from build123d import *

# Parameters (mm, degrees)
F0_R     = 1.25
F1_DEPTH = 0.55
F2_R     = 0.695
F3_DEPTH = 7.3
F4_W     = 0.45
F4_H     = 0.45
F4_H_2   = 0.575
F4_W_2   = 0.575
F5_DEPTH = 0.3
F6_R     = 0.2


with BuildPart() as f1:
    # F0 (on Top) → F1 (new body)
    with BuildSketch(Plane.XY):
        Circle(F0_R)
    extrude(amount=F1_DEPTH)

    # F2 (on face) → F3 (join)
    with BuildSketch(Plane(origin=(0, 0, 0), x_dir=(1, 0, 0), z_dir=(0, 0, -1))):
        Circle(F2_R)
    extrude(amount=F3_DEPTH)

    # F4 (on face) → F5 (cut)
    with BuildSketch(Plane.XY.offset(0.55)):
        Rectangle(F4_W, F4_H)
        with Locations((0, 0.5125)):
            Rectangle(F4_W, F4_H_2)
        with Locations((-0.5125, 0)):
            Rectangle(F4_W_2, F4_H)
        with Locations((0, -0.5125)):
            Rectangle(F4_W, F4_H_2)
        with Locations((0.5125, 0)):
            Rectangle(F4_W_2, F4_H)
    extrude(amount=-F5_DEPTH, mode=Mode.SUBTRACT)

    # F6
    f6_edges = [f1.edges().sort_by_distance(p)[0] for p in [
        (-1.25, 0, 0.55),
        (-1.25, 0, 0),
    ]]
    fillet(f6_edges, radius=F6_R)


solid = f1.part
CAD build for the part. Positions are in the model's coordinates, mm. Round coordinates to 2 decimals unless told otherwise and drop trailing zeros. Write each loop counter-clockwise with the first axis right and the second up, starting at its lowest first coordinate (ties: lowest second). Pieces come first, ordered by that corner, then holes.
(1) Slice it at C-C, the plane z = -2.5. Write the cut outline in (x, y) (3 decimals).
(2) Slice it at A-A, the plane y = 0. Write the cut outline in (x, z) (3 decimals), and give its area (3 significant figures).
(3) Drop flat-ended pins along their axis: P1, Ø1, axis at y = 1, z = -5.5, coming from the -X side; P2, Ø1, axis at y = 0, z = -2.5, coming from the -X side (3 decimals). Give the stop position or say it passes through.
(4) Probe line 1 along Z through (x, y) = (0.05, -0.05); line 2 along Y through (x, z) = (0, -6) (3 decimals); line 3 along Z through (x, y) = (-0.5, -0.7). List the from-to ranges inside material, lowest first.
(5) Mould opens along X. For faces 1 (the face through (0.5, -0.5, 0.55)), 2 (the face through (-0.552, 0.423, -3.599)), 3 (the face through (0, 0, 0.25)) say: pulls with the +X half, pulls with the -X half, needs draft (parallel to the pull), parting line crosses it, or undercut.
From the geometry:
1. outline: circle Ø1.39 at (0, 0)
2. outline: (-1.25, 0.2) arc R0.2 ccw to (-1.05, 0) - (-0.695, 0) - (-0.695, -7.3) - (0.695, -7.3) - (0.695, 0) - (1.05, 0) arc R0.2 ccw to (1.25, 0.2) - (1.25, 0.35) arc R0.2 ccw to (1.05, 0.55) - (0.8, 0.55) - (0.8, 0.25) - (-0.8, 0.25) - (-0.8, 0.55) - (-1.05, 0.55) arc R0.2 ccw to (-1.25, 0.35) - close
2. area: 11.0 mm2
3. P1: stops at x = -0.48
3. P2: stops at x = -0.695
4. line 1: z = -7.3 to 0.25
4. line 2: y = -0.695 to 0.695
4. line 3: z = 0 to 0.55
5. face 1: needs draft
5. face 2: parting line crosses it
5. face 3: undercut
